Work out the finished part from the listing and answer in its coordinate system (mm). Coordinates: 2 decimals unless noted, no trailing zeros. Loops run counter-clockwise (first coordinate to the right, second up) from the corner with the lowest first, then second, coordinate; pieces in that order, holes last. Notation, with made-up numbers: (33.5, -16.5) -> (91.5, -16.5) arc R24 cw to (91.5, -0.5) -> close; hole circle Ø10 at (30.25, -10). An arc over 180 degrees is marked (long way). Use a Markdown table: item, result. Add a question column.
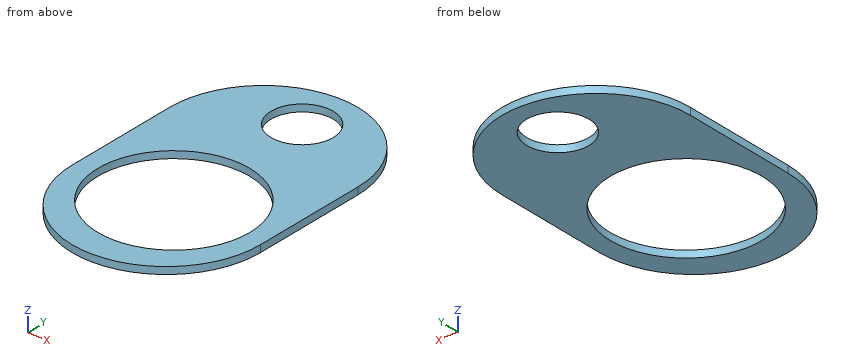
```python
from build123d import *

# Parameters (mm, degrees)
FASTENER_BODY_DEPTH = 1.17602
CUT_EXTRUDE2_REACH  = 49.138
SKETCH3_R           = 5.207
SKETCH3_R_2         = 12.7


with BuildPart() as part:
    # Sketch2 → Fastener Body (new body)
    with BuildSketch(Plane.XY):
        with BuildLine():
            Line((0, 0), (0, 19.304))
            ThreePointArc((0, 19.304), (15.748, 35.052), (31.496, 19.304))
            Line((31.496, 19.304), (31.496, 0))
            ThreePointArc((31.496, 0), (15.748, -15.748), (0, 0))
        make_face()
    extrude(amount=-FASTENER_BODY_DEPTH)

    # Sketch3 → Cut-Extrude2 (cut, up to next)
    with BuildSketch(Plane.XY, mode=Mode.PRIVATE) as cut_extrude2_sk1:
        with Locations((15.748, 26.902177492)):
            Circle(SKETCH3_R)
    cut_extrude2_tool1 = extrude(cut_extrude2_sk1.sketch, amount=-CUT_EXTRUDE2_REACH, mode=Mode.PRIVATE) & part.part
    # Sketch3 → Cut-Extrude2 (cut, up to next)
    with BuildSketch(Plane.XY, mode=Mode.PRIVATE) as cut_extrude2_sk2:
        with Locations((15.748, 1.502177492)):
            Circle(SKETCH3_R_2)
    cut_extrude2_tool2 = extrude(cut_extrude2_sk2.sketch, amount=-CUT_EXTRUDE2_REACH, mode=Mode.PRIVATE) & part.part
    add(cut_extrude2_tool1.solids().sort_by_distance((15.748, 26.902177, 0))[0], mode=Mode.SUBTRACT)
    add(cut_extrude2_tool2.solids().sort_by_distance((15.748, 1.502177, 0))[0], mode=Mode.SUBTRACT)


solid = part.part
```
Item 1: Section A-A (y = 24) is taken. Determine the outline of the cut face in (x, z), then the cut area to 3 significant figures.
Item 2: Section B-B (x = 18) is taken. Determine the outline of the cut face in (y, z), then the cut area to 3 significant figures.
Item 3: Given pin 1 (16.5 mm diameter, centred on x = 15.75, y = 26.9, fed in from -Z), flat-ended and moving along its own axis, determine where the tip first touches the part or whether it passes through.
Item 4: Section D-D (z = -0.2) is taken. Determine the outline of the cut face in (x, y) (3 decimals).
Item 5: Find the intervals of material crossed by probe 1 along Y at (x, z) = (16, -0.65); probe 2 along Y at (x, z) = (11, -0.5); probe 3 along X at (y, z) = (1, -1), in increasing order.
Item 6: Section C-C (x = 25.5) is taken. Determine the outline of the cut face in (y, z), then the cut area to 4 significant figures.
Output:
| question | item | result |
|---|---|---|
| 1 | outline | (0.72, -1.18) -> (11.42, -1.18) -> (11.42, 0) -> (0.72, 0) -> close; (20.07, -1.18) -> (30.78, -1.18) -> (30.78, 0) -> (20.07, 0) -> close |
| 1 | area | 25.2 mm2 |
| 2 | outline | (-15.59, -1.18) -> (-11, -1.18) -> (-11, 0) -> (-15.59, 0) -> close; (14, -1.18) -> (22.21, -1.18) -> (22.21, 0) -> (14, 0) -> close; (31.6, -1.18) -> (34.89, -1.18) -> (34.89, 0) -> (31.6, 0) -> close |
| 2 | area | 18.9 mm2 |
| 3 | pin 1 | stops at z = -1.18 |
| 4 | outline | (0, 0) arc R15.748 ccw to (31.496, 0) -> (31.496, 19.304) arc R15.748 ccw to (0, 19.304) -> close; hole circle Ø25.4 at (15.748, 1.502); hole circle Ø10.414 at (15.748, 26.902) |
| 5 | probe 1 | y = -15.75 to -11.2, 14.2 to 21.7, 32.1 to 35.05 |
| 5 | probe 2 | y = -15.02 to -10.28, 13.28 to 24.76, 29.04 to 34.32 |
| 5 | probe 3 | x = 0 to 3.06, 28.44 to 31.5 |
| 6 | outline | (-12.37, -1.18) -> (-6.63, -1.18) -> (-6.63, 0) -> (-12.37, 0) -> close; (9.64, -1.18) -> (31.67, -1.18) -> (31.67, 0) -> (9.64, 0) -> close |
| 6 | area | 32.65 mm2 |
